For this review, take the finished solid that the model builds, in its own axes (mm). A direction names the side the tool comes from. Coordinates: 2 decimals unless noted, no trailing zeros. Order: outer loops, then holes, each group sorted by start corner. A loop starts at its lowest first (then second) coordinate and runs counter-clockwise, first axis right, second up. Notation, with made-up numbers: M 67.25,76.5 L 92.25,76.5 A7 cw 92.25,87.5 Z; hole C 34,22.5 d1. An arc over 180 degrees is marked long. Use CSV: the item, a comma, the result in double quotes.
Autodesk Inventor part; units mm, degrees
ref_plane "YZ Plane" through (0, 0, 0) normal (1, 0, 0) x (0, 1, 0)
ref_plane "XZ Plane" through (0, 0, 0) normal (0, 1, 0) x (-1, 0, 0)
ref_plane "XY Plane" through (0, 0, 0) normal (0, 0, 1) x (1, 0, 0)
sketch "スケッチ1" plane through (0, 0, 0) normal (0, 0, 1) x (1, 0, 0)
  circle A0 centre (68.955, 78.0364) radius 1.25
  arc A1 (82.2061, 79.4541) -> (58.0365, 100.3664) centre (53.5087, 70.7101) ccw
  arc A2 (58.0365, 100.3664) -> (49.826, 85.6345) centre (56.6782, 91.4695) ccw
  line L0 (78.21, 52.3031) -> (49.826, 85.6345)
  line L1 (85.7362, 40.2517) -> (78.21, 52.3031)
  arc A3 (85.7362, 40.2517) -> (86.8285, 38.9062) centre (91.6947, 43.9728) ccw
  line L2 (104.8592, 21.5887) -> (86.8285, 38.9062)
  arc A4 (104.8592, 21.5887) -> (116.6904, 27.5718) centre (109.7254, 26.6553) ccw
  line L3 (114.602, 43.4428) -> (116.6904, 27.5718)
  arc A5 (114.602, 43.4428) -> (113.6245, 46.2008) centre (107.6371, 42.5263) ccw
  line L4 (100.6394, 67.3594) -> (113.6245, 46.2008)
  arc A6 (100.6394, 67.3594) -> (89.5888, 73.7904) centre (89.1334, 60.2981) ccw
  arc A7 (82.2061, 79.4541) -> (89.5888, 73.7904) centre (89.8587, 81.7859) ccw
  circle A8 centre (89.1334, 60.2981) radius 8.525
  circle A9 centre (109.7254, 26.6553) radius 3.025
  circle A10 centre (107.6371, 42.5263) radius 3.025
  circle A11 centre (91.6947, 43.9728) radius 3.025
  circle A12 centre (56.6782, 91.4695) radius 1.25
  circle A13 centre (109.7254, 26.6553) radius 7.025
  circle A14 centre (91.6947, 43.9728) radius 7.025
  circle A15 centre (107.6371, 42.5263) radius 7.025
  line L5 (92.3295, 50.9691) -> (108.2718, 49.5226)
  point P0 (0, 0)
  point P1 (0, 0)
extrude "押し出し1" add sketch "スケッチ1" against normal blind 4 contours A5 A15 | A14 A3 | L3 A13 L2 A14 L5 A15 | A4 A13
sketch "スケッチ2" plane through (0, 0, 0) normal (0, 0, 1) x (1, 0, 0)
  arc A0 (104.8592, 21.5887) -> (116.6904, 27.5718) centre (109.7254, 26.6553) ccw
  line L0 (116.6904, 27.5718) -> (114.602, 43.4428)
  arc A1 (114.602, 43.4428) -> (108.2718, 49.5226) centre (107.6371, 42.5263) ccw
  line L1 (108.2718, 49.5226) -> (92.3295, 50.9691)
  arc A2 (92.3295, 50.9691) -> (86.8285, 38.9062) centre (91.6947, 43.9728) ccw
  line L2 (86.8285, 38.9062) -> (104.8592, 21.5887)
  circle A3 centre (107.6371, 42.5263) radius 3.025
  circle A4 centre (109.7254, 26.6553) radius 3.025
  circle A5 centre (91.6947, 43.9728) radius 3.025
  line L3 (108.2718, 49.5226) -> (92.3295, 50.9691)
  circle A6 centre (109.7254, 26.6553) radius 3.025
  arc A7 (104.8592, 21.5887) -> (116.6904, 27.5718) centre (109.7254, 26.6553) ccw
  point P0 (0, 0)
sketch "スケッチ3" plane through (0, 0, 0) normal (0, 0, 1) x (1, 0, 0)
  arc A0 (104.8592, 21.5887) -> (116.6904, 27.5718) centre (109.7254, 26.6553) ccw
  line L0 (116.6904, 27.5718) -> (114.602, 43.4428)
  arc A1 (114.602, 43.4428) -> (108.2718, 49.5226) centre (107.6371, 42.5263) ccw
  line L1 (108.2718, 49.5226) -> (92.3295, 50.9691)
  arc A2 (92.3295, 50.9691) -> (86.8285, 38.9062) centre (91.6947, 43.9728) ccw
  line L2 (86.8285, 38.9062) -> (104.8592, 21.5887)
  circle A3 centre (107.6371, 42.5263) radius 3.025
  circle A4 centre (109.7254, 26.6553) radius 3.025
  circle A5 centre (91.6947, 43.9728) radius 3.025
  arc A6 (106.9373, 23.7524) -> (113.716, 27.1804) centre (109.7254, 26.6553) ccw
  line L3 (113.716, 27.1804) -> (111.6277, 43.0514)
  arc A7 (111.6277, 43.0514) -> (108.0008, 46.5349) centre (107.6371, 42.5263) ccw
  line L4 (108.0008, 46.5349) -> (92.0584, 47.9813)
  arc A8 (92.0584, 47.9813) -> (88.9066, 41.0699) centre (91.6947, 43.9728) ccw
  line L5 (88.9066, 41.0699) -> (106.9373, 23.7524)
  line L6 (104.8592, 21.5887) -> (86.8285, 38.9062)
  circle A9 centre (91.6947, 43.9728) radius 7.025
  line L7 (114.602, 43.4428) -> (116.6904, 27.5718)
  circle A10 centre (107.6371, 42.5263) radius 7.025
  circle A11 centre (109.7254, 26.6553) radius 7.025
  point P0 (0, 0)
  point P1 (102.7848, 27.7407)
  point P2 (112.9649, 32.8888)
  point P3 (112.3788, 37.343)
  point P4 (102.2667, 47.0551)
  point P5 (97.7925, 47.4611)
  point P6 (93.0592, 37.0816)
  dimension "d2" = 3
extrude "押し出し2" cut sketch "スケッチ3" against normal blind 3.5 contours L5 A9 L4 A10 L3 A11
sketch "スケッチ4" plane through (0, 0, 0) normal (0, 0, 1) x (1, 0, 0)
  line L0 (112.3788, 37.343) -> (112.9649, 32.8888)
  arc A0 (112.9649, 32.8888) -> (102.7848, 27.7407) centre (109.7254, 26.6553) ccw
  line L1 (102.7848, 27.7407) -> (93.0592, 37.0816)
  arc A1 (93.0592, 37.0816) -> (97.7925, 47.4611) centre (91.6947, 43.9728) ccw
  line L2 (97.7925, 47.4611) -> (102.2667, 47.0551)
  arc A2 (102.2667, 47.0551) -> (112.3788, 37.343) centre (107.6371, 42.5263) ccw
  arc A3 (104.8592, 21.5887) -> (116.6904, 27.5718) centre (109.7254, 26.6553) ccw
  line L3 (116.6904, 27.5718) -> (114.602, 43.4428)
  arc A4 (114.602, 43.4428) -> (108.2718, 49.5226) centre (107.6371, 42.5263) ccw
  line L4 (108.2718, 49.5226) -> (92.3295, 50.9691)
  arc A5 (92.3295, 50.9691) -> (86.8285, 38.9062) centre (91.6947, 43.9728) ccw
  line L5 (86.8285, 38.9062) -> (104.8592, 21.5887)
  circle A6 centre (107.6371, 42.5263) radius 3.025
  circle A7 centre (109.7254, 26.6553) radius 3.025
  circle A8 centre (91.6947, 43.9728) radius 3.025
  arc A9 (102.2667, 47.0551) -> (112.3788, 37.343) centre (107.6371, 42.5263) ccw
  line L6 (91.6947, 43.9728) -> (107.6371, 42.5263) construction
  line L7 (91.6722, 43.7238) -> (107.6145, 42.2774)
  line L8 (107.6597, 42.7753) -> (91.7173, 44.2218)
  arc A10 (91.7173, 44.2218) -> (91.6722, 43.7238) centre (91.6947, 43.9728) ccw
  arc A11 (107.6145, 42.2774) -> (107.6597, 42.7753) centre (107.6371, 42.5263) ccw
  line L9 (107.6371, 42.5263) -> (109.7254, 26.6553) construction
  line L10 (107.3892, 42.4937) -> (109.4776, 26.6227)
  line L11 (109.9733, 26.688) -> (107.8849, 42.559)
  arc A12 (107.8849, 42.559) -> (107.3892, 42.4937) centre (107.6371, 42.5263) ccw
  arc A13 (109.4776, 26.6227) -> (109.9733, 26.688) centre (109.7254, 26.6553) ccw
  point P0 (0, 0)
  point P1 (99.6659, 43.2496)
  point P2 (108.6812, 34.5908)
  point P3 (109.0574, 33.6485)
  point P4 (108.8008, 35.5984)
  point P5 (108.3051, 35.5332)
  point P6 (108.5617, 33.5833)
  point P7 (100.6678, 43.4097)
  point P8 (98.7092, 43.5874)
  point P9 (98.664, 43.0895)
  point P10 (100.6227, 42.9117)
  dimension "d9" = 0.5
  dimension "d10" = 0.5
extrude "押し出し3" add sketch "スケッチ4" against normal blind 4 contours L11 A0 L10 A2 | L7 A1 L8 A2
fillet "フィレット1" radius 1 14 edges at (97.7925, 47.4611, -1.75) (102.2667, 47.0551, -1.75) (98.7092, 43.5874, -1.75) (98.664, 43.0895, -1.75) (100.6678, 43.4097, -1.75) (100.6227, 42.9117, -1.75) (93.0592, 37.0816, -1.75) (112.3788, 37.343, -1.75) (112.9649, 32.8888, -1.75) (108.8008, 35.5984, -1.75) (108.3051, 35.5332, -1.75) (109.0574, 33.6485, -1.75) (108.5617, 33.5833, -1.75) (102.7848, 27.7407, -1.75)
properties part number "アーム 中間節 中詰め" material "ABS プラスチック"
Item 1: Clearance check with flat-ended pins moving along their axes: pin 1 Ø5 at (x, y) = (91.69, 43.97) entering from -Z; pin 2 Ø1 at (x, z) = (105.5, -3) entering from +Y; pin 3 Ø7 at (x, y) = (107.64, 42.53) entering from -Z; pin 4 Ø0.9 at (x, y) = (100, 45.5) entering from +Z. State where each tip first meets the part, or that it passes through.
Solutions:
pin 1,"through"
pin 2,"y = 49.82"
pin 3,"z = -4"
pin 4,"z = -3.5"
Item 2: Add section C-C on z = -0.5. State how many separate pieces and enclosed holes the cut face has, and give its area (3 significant figures).
Solutions:
separate pieces,"1"
enclosed holes,"6"
area,"484 mm^2"
Item 3: Add section A-A on y = 24. State the section outline as (x, z) points, and give its area (3 significant figures).
Solutions:
outline,"M 102.35,-4 L 108.28,-4 L 108.28,0 L 102.35,0 Z; M 111.17,-4 L 116.23,-4 L 116.23,0 L 111.17,0 Z"
area,"43.9 mm^2"
Item 4: For faces 5 (the face through (114.265, 44.854, -1.972)), 6 (the face through (112.039, 36.453, -1.774)), list the 3-axis set-ups (+Z, -Z, +X, -X, +Y, -Y) from which the entire face can be reached by the end or side of a thin tool; tool diameter is ignored.
Solutions:
face 5,"+Z, -Z, +X, +Y"
face 6,"+Z"
Item 5: To check wall thickness, follow line 1 along X through (y, z) = (46, -1.85); line 2 along Y through (x, z) = (100.5, -2); line 3 along Y through (x, z) = (108, -3.35). State the ranges of each line that lie inside material, in increasing order. Write a range as [from, to].
Solutions:
line 1,"[84.97, 89.45], [93.94, 98.42], [101.49, 113.74]"
line 2,"[25.78, 29.94], [42.49, 43.72], [47.22, 50.23]"
line 3,"[19.85, 24.17], [29.14, 33.52], [35.33, 39.52], [45.53, 49.55]"
Item 6: Add section D-D on y = 28. State the section outline as (x, z) points.
Solutions:
outline,"M 98.18,-4 L 107.02,-4 L 107.02,0 L 98.18,0 Z; M 112.44,-4 L 116.63,-4 L 116.63,0 L 112.44,0 Z"
Item 7: Add section B-B on y = 33. State the section outline as (x, z) points, and give its area (3 significant figures).
Solutions:
outline,"M 92.98,-4 L 115.98,-4 L 115.98,0 L 106.71,0 L 106.71,-3.5 L 97.31,-3.5 L 97.31,0 L 92.98,0 Z"
area,"59.1 mm^2"
Item 8: Draft analysis for pull direction X (two halves, no side actions). For faces 1 (the face through (100.189, 50.256, -1.972)), 2 (the face through (101.38, 46.7, -1.77)), 3 (the face through (111, 35, -3.5)), 4 (the face through (104, 39, -4)), state which applies: released by +X, released by -X, zero draft, split by the parting line, or undercut.
Solutions:
face 1,"released by +X"
face 2,"undercut"
face 3,"undercut"
face 4,"zero draft"
